Input: part model. Units: mm. Frame: model coordinates. Face numbers are marked on the shaded views. Give positions to 0.01 mm unless a question says otherwise; leave off trailing zeros. Loops run counter-clockwise (first coordinate to the right, second up) from the corner with the lowest first, then second, coordinate; pieces in that order, holes last.
from build123d import *

# Parameters (mm, degrees)
SKETCH_W               = 15
SKETCH_H               = 95.5
PAD_DEPTH              = 10
SKETCH001_W            = 9.1
SKETCH001_H            = 9.1
POCKET_DEPTH           = 0.001
POCKET_DEPTH_BACK      = 10.001
LINEARPATTERN_COUNT    = 7
LINEARPATTERN_PITCH    = 13.2
SKETCH002_W            = 11.5
SKETCH002_H            = 11.5
POCKET001_DEPTH        = 1
LINEARPATTERN001_COUNT = 7
LINEARPATTERN001_PITCH = 13.2
CHAMFER_SIZE           = 2
FILLET_R               = 1


with BuildPart() as part:
    # Sketch → Pad (new body)
    with BuildSketch(Plane.XY):
        with Locations((7.5, 47.75)):
            Rectangle(SKETCH_W, SKETCH_H)
    extrude(amount=PAD_DEPTH)

    # Sketch001 → Pocket (cut, two sides)
    with BuildSketch(Plane.XY) as pocket_sk:
        with Locations((7.5, 7.55)):
            Rectangle(SKETCH001_W, SKETCH001_H)
    pocket = extrude(amount=-POCKET_DEPTH, mode=Mode.SUBTRACT) + extrude(pocket_sk.sketch, amount=POCKET_DEPTH_BACK, mode=Mode.SUBTRACT)

    # LinearPattern: Pocket ×7
    with Locations(*[(0, i * LINEARPATTERN_PITCH, 0) for i in range(1, LINEARPATTERN_COUNT)]):
        add(pocket, mode=Mode.SUBTRACT)

    # Sketch002 → Pocket001 (cut)
    with BuildSketch(Plane.XY):
        with Locations((7.5, 7.55)):
            Rectangle(SKETCH002_W, SKETCH002_H)
    pocket001 = extrude(amount=POCKET001_DEPTH, mode=Mode.SUBTRACT)

    # LinearPattern001: Pocket001 ×7
    with Locations(*[(0, i * LINEARPATTERN001_PITCH, 0) for i in range(1, LINEARPATTERN001_COUNT)]):
        add(pocket001, mode=Mode.SUBTRACT)

    # Chamfer
    chamfer_edges = [part.edges().sort_by_distance(p)[0] for p in [
        (12.05, 7.55, 10),
        (7.5, 3, 10),
        (2.95, 7.55, 10),
        (7.5, 12.1, 10),
        (2.95, 20.75, 10),
        (7.5, 16.2, 10),
        (7.5, 25.3, 10),
        (12.05, 20.75, 10),
        (7.5, 29.4, 10),
        (2.95, 33.95, 10),
        (7.5, 38.5, 10),
        (12.05, 33.95, 10),
        (7.5, 42.6, 10),
        (2.95, 47.15, 10),
        (7.5, 51.7, 10),
        (12.05, 47.15, 10),
        (2.95, 60.35, 10),
        (7.5, 55.8, 10),
        (7.5, 64.9, 10),
        (12.05, 60.35, 10),
        (7.5, 69, 10),
        (2.95, 73.55, 10),
        (7.5, 78.1, 10),
        (12.05, 73.55, 10),
        (7.5, 82.2, 10),
        (2.95, 86.75, 10),
        (7.5, 91.3, 10),
        (12.05, 86.75, 10),
    ]]
    chamfer(chamfer_edges, length=CHAMFER_SIZE)

    # Fillet
    fillet_edges = [part.edges().sort_by_distance(p)[0] for p in [
        (15, 0, 5),
        (0, 0, 5),
        (15, 95.5, 5),
        (0, 95.5, 5),
    ]]
    fillet(fillet_edges, radius=FILLET_R)


solid = part.part
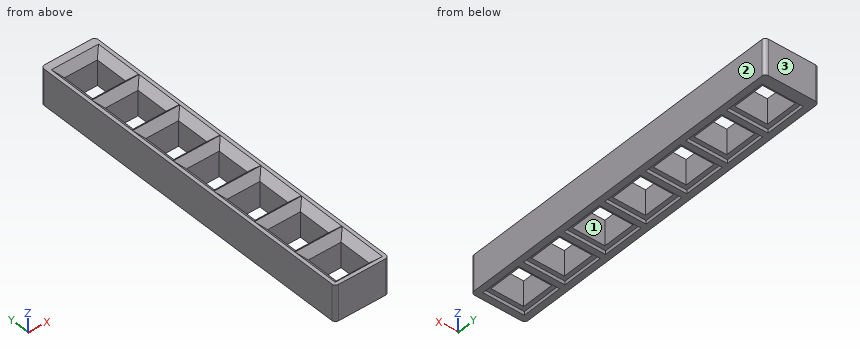
(1) Mould query, pull axis Y, two halves, no side actions, for the marked faces 1, 2 and 3. Classes: +Y half, -Y half, draft (parallel to the pull), parting line (faces both ways), or undercut.
Values follow:
face 1: undercut
face 2: draft
face 3: +Y half
(2) Cut plane A-A (y = 20.5). Return the cut outline in (x, z).
Values follow:
outline: (0, 0) - (1.75, 0) - (1.75, 1) - (2.95, 1) - (2.95, 8) - (0.95, 10) - (0, 10) - close; (12.05, 1) - (13.25, 1) - (13.25, 0) - (15, 0) - (15, 10) - (14.05, 10) - (12.05, 8) - close
(3) Cut plane B-B (x = 5). Count the separate pieces of the cut face and the enclosed holes in it, and give its area (3 significant figures).
Values follow:
separate pieces: 8
enclosed holes: 0
area: 273 mm2
(4) Ray query, probe 1 along X at (y, z) = (60.5, 4); probe 2 along X at (y, z) = (30.5, 0.5); probe 3 along Z at (x, y) = (11.25, 79.5). Return the intervals inside material, ascending.
Values follow:
probe 1: x = 0 to 2.95, 12.05 to 15
probe 2: x = 0 to 1.75, 13.25 to 15
probe 3: z = 0 to 9.4
